Here's how the part is built. I have some questions about the finished solid (model axes, mm). Round coordinates to 2 decimals unless told otherwise and drop trailing zeros. Write each loop counter-clockwise with the first axis right and the second up, starting at its lowest first coordinate (ties: lowest second). Pieces come first, ordered by that corner, then holes. Notation, with made-up numbers: (-32, 75.5) -> (-28, 75.5) arc R8 cw to (-28, 86.5) -> close; hole circle Ø5 at (53, 33.5). An arc over 180 degrees is marked (long way). Answer as CSV lines item,"result".
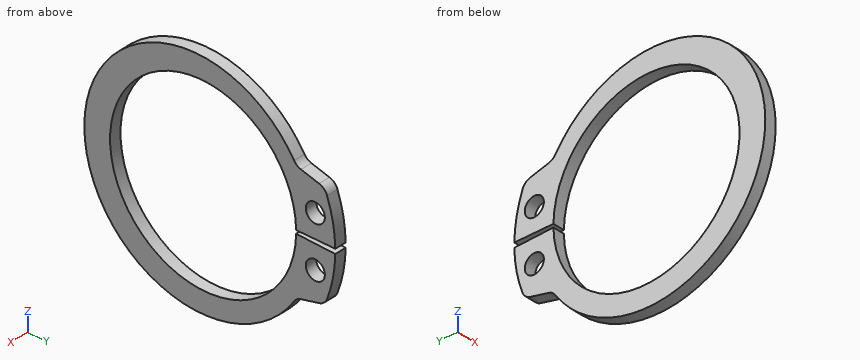
from build123d import *

# Parameters (mm, degrees)
SKETCH1_R           = 1
BOSS_EXTRUDE1_DEPTH = 1.2


with BuildPart() as part:
    # Sketch1 → Boss-Extrude1 (new body)
    with BuildSketch(Plane(origin=(-0.6, 0, 0), x_dir=(0, -1, 0), z_dir=(-1, 0, 0))):
        with BuildLine():
            Line((-10.254517122, 6.020654884), (-12.157117236, 5.546283398))
            ThreePointArc((-12.157117236, 5.546283398), (-12.667686664, 5.275571693), (-12.992516349, 4.797605541))
            ThreePointArc((-12.992516349, 4.797605541), (-13.612159776, 2.555700733), (-13.847890578, 0.241715829))
            Line((-13.847890578, 0.241715829), (-9.748515028, 0.170160963))
            ThreePointArc((-9.748515028, 0.170160963), (9.75, 0), (-9.748515028, -0.170160963))
            Line((-9.748515028, -0.170160963), (-13.847890578, -0.241715829))
            ThreePointArc((-13.847890578, -0.241715829), (-13.612159776, -2.555700733), (-12.992516349, -4.797605541))
            ThreePointArc((-12.992516349, -4.797605541), (-12.667686664, -5.275571693), (-12.157117236, -5.546283398))
            Line((-12.157117236, -5.546283398), (-10.254517122, -6.020654884))
            ThreePointArc((-10.254517122, -6.020654884), (-9.848654609, -6.207590185), (-9.539322273, -6.530053659))
            ThreePointArc((-9.539322273, -6.530053659), (12.45, 0), (-9.539322273, 6.530053659))
            ThreePointArc((-9.539322273, 6.530053659), (-9.848654609, 6.207590185), (-10.254517122, 6.020654884))
        make_face()
        with Locations((-11.755399891, -2.658115574)):
            Circle(SKETCH1_R, mode=Mode.SUBTRACT)
        with Locations((-11.755399891, 2.658115574)):
            Circle(SKETCH1_R, mode=Mode.SUBTRACT)
    extrude(amount=-BOSS_EXTRUDE1_DEPTH)


solid = part.part
Item 1: I need wall thicknesses on L1, parallel to Y at x = 0.05, z = 3; L2, parallel to Y at x = -0.1, z = 0; L3, parallel to Z at x = -0.4, y = -6.5. Which ranges of each line are inside material? Lowest first, please.
Results found:
L1,"y = -12.07 to -9.28, 9.28 to 10.82, 12.7 to 13.52"
L2,"y = -12.45 to -9.75"
L3,"z = -10.34 to -7.27, 7.27 to 10.34"
Item 2: Suppose I cut it at C-C, the plane x = 0.35. List the corners of the cut face in (y, z) for me (3 decimals), then the cut area to 3 significant figures.
Results found:
outline,"(9.539, -6.53) arc R1.2 cw to (10.255, -6.021) -> (12.157, -5.546) arc R1.2 ccw to (12.993, -4.798) arc R13.85 ccw to (13.848, -0.242) -> (9.749, -0.17) arc R9.75 cw (long way) to (9.749, 0.17) -> (13.848, 0.242) arc R13.85 ccw to (12.993, 4.798) arc R1.2 ccw to (12.157, 5.546) -> (10.255, 6.021) arc R1.2 cw to (9.539, 6.53) arc R11.964 ccw (long way) to start; hole circle Ø2 at (11.755, -2.658); hole circle Ø2 at (11.755, 2.658)"
area,"171 mm²"
Item 3: Suppose I cut it at A-A, the plane z = 8.5. List the corners of the cut face in (x, y) for me, then the cut area to 3 significant figures.
Results found:
outline,"(-0.6, -8.91) -> (0.6, -8.91) -> (0.6, -4.78) -> (-0.6, -4.78) -> close; (-0.6, 4.78) -> (0.6, 4.78) -> (0.6, 7.93) -> (-0.6, 7.93) -> close"
area,"8.74 mm²"
Item 4: Suppose I cut it at B-B, the plane y = 5.25. List the corners of the cut face in (x, z) for me, then the cut area to 3 significant figures.
Results found:
outline,"(-0.6, -10.5) -> (0.6, -10.5) -> (0.6, -8.22) -> (-0.6, -8.22) -> close; (-0.6, 8.22) -> (0.6, 8.22) -> (0.6, 10.5) -> (-0.6, 10.5) -> close"
area,"5.48 mm²"
